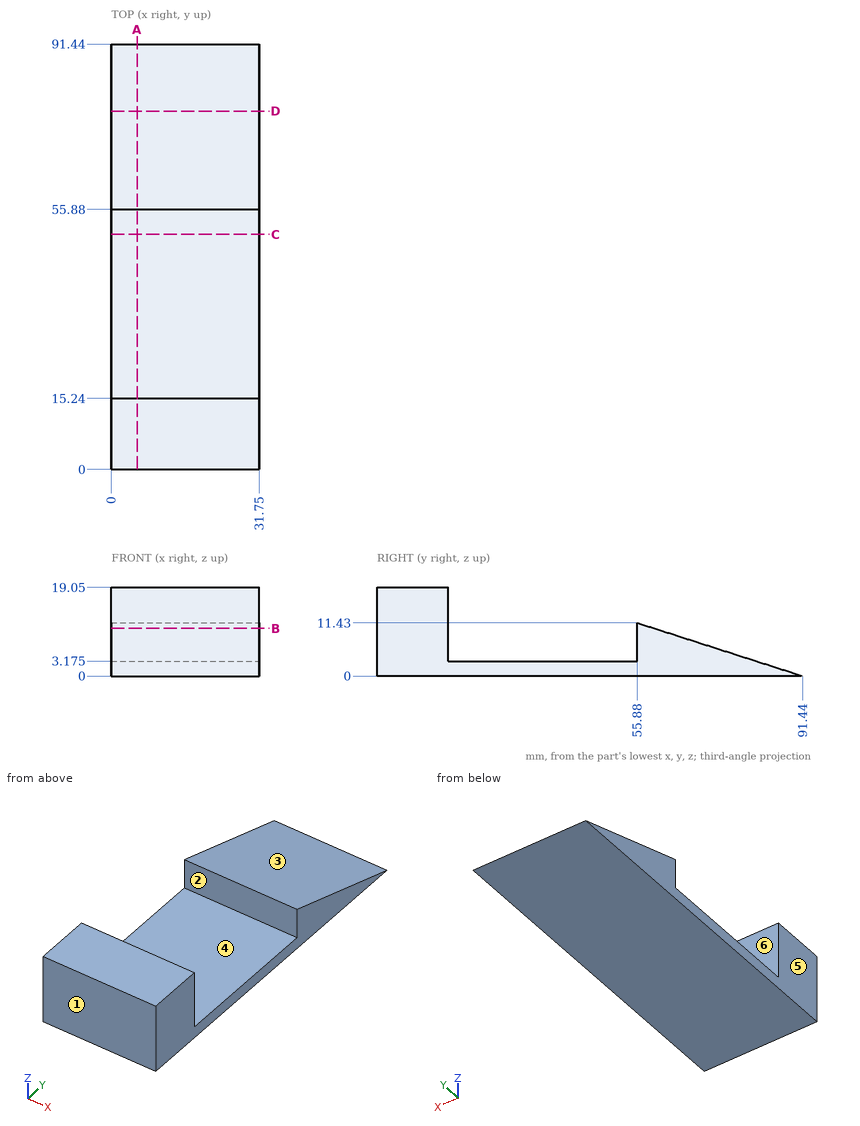
Geometry: see drawing. Coordinates: mm, zero at the bounding-box minimum. A direction names the side the tool comes from. Give positions to 0.01 mm unless a question says otherwise; leave off trailing zeros. Order: outer loops, then holes, each group sorted by start corner. A loop starts at its lowest first (then second) coordinate and runs counter-clockwise, first axis right, second up. Notation, with made-up numbers: M -11,88.25 L 6,88.25 A23 ccw 6,107.25 Z; hole C 1,31 d5. An arc over 180 degrees is marked long. Answer as a JSON object with one key per item and string values.
1. Pull-direction query (Y, two-part tool) for the marked faces 1, 2, 3 and 4; classes: +Y half, -Y half, draft (parallel to the pull), parting line (faces both ways), or undercut.
Result sheet:
{"face 1": "-Y half", "face 2": "undercut", "face 3": "+Y half", "face 4": "undercut"}
2. Reachability of the marked faces 5 and 6 from +Z, -Z, +X, -X, +Y, -Y: full face, straight path, thin tool, end or side. Return the list, or none.
Result sheet:
{"face 5": "+Z, -Z, -X, +Y, -Y", "face 6": "+Z, +X, -X"}
3. Ray query, line 1 (Y direction, x = 30.5, z = 16); line 2 (Z direction, x = 21.5, y = 50) (3 decimals); line 3 (Z direction, x = 28.5, y = 57.5). Return the intervals inside material, ascending. Write a range as [from, to].
Result sheet:
{"line 1": "[0, 15.24]", "line 2": "[0, 3.175]", "line 3": "[0, 10.91]"}
4. First-contact query: P1, Ø6, axis at x = 26, y = 40, coming from the +Z side (3 decimals). Flat tip, straight axial feed; report the tip coordinate or a pass-through.
Result sheet:
{"P1": "z = 3.175"}
5. Cut plane B-B, the plane z = 10.25. Output: boundary loops of the cut face in (x, y), and give its area (3 significant figures).
Result sheet:
{"outline": "M 0,0 L 31.75,0 L 31.75,15.24 L 0,15.24 Z; M 0,55.88 L 31.75,55.88 L 31.75,59.55 L 0,59.55 Z", "area": "600 mm²"}
6. Cut plane A-A, the plane x = 5.5. Output: boundary loops of the cut face in (y, z) (3 decimals), and give its area (3 significant figures).
Result sheet:
{"outline": "M 0,0 L 91.44,0 L 55.88,11.43 L 55.88,3.175 L 15.24,3.175 L 15.24,19.05 L 0,19.05 Z", "area": "623 mm²"}
7. Cut plane D-D, the plane y = 77. Output: boundary loops of the cut face in (x, z), and give its area (3 significant figures).
Result sheet:
{"outline": "M 0,0 L 31.75,0 L 31.75,4.64 L 0,4.64 Z", "area": "147 mm²"}
8. Cut plane C-C, the plane y = 50.5. Output: boundary loops of the cut face in (x, z) (3 decimals).
Result sheet:
{"outline": "M 0,0 L 31.75,0 L 31.75,3.175 L 0,3.175 Z"}
